Build history of the part. All positions in model axes, mm. A direction names the side the tool comes from. Round coordinates to 2 decimals unless told otherwise and drop trailing zeros. Order: outer loops, then holes, each group sorted by start corner. A loop starts at its lowest first (then second) coordinate and runs counter-clockwise, first axis right, second up. Notation, with made-up numbers: M 19.5,67.5 L 78.5,67.5 A21 cw 78.5,88.5 Z; hole C 36.25,58.5 d5. An arc over 180 degrees is marked long. Use CSV: the item, a comma, the result in double quotes.
from build123d import *

# Parameters (mm, degrees)
F1_DEPTH = 5
F2_R     = 2
F3_R     = 2.224598
F4_DEPTH = 35.001


with BuildPart() as f1:
    # F0 (on Front) → F1 (new body, symmetric)
    with BuildSketch(Plane.XZ):
        Polygon((53.206599, 9.36247), (53.206599, 39.36247), (54.706599, 39.36247), (54.706599, 29.36247), (59.706599, 29.36247), (59.706599, 44.36247), (48.206599, 44.36247), (48.206599, 9.36247), align=None)
    extrude(amount=F1_DEPTH, both=True)

    # F2
    f2_edges = [f1.edges().sort_by_distance(p)[0] for p in [
        (59.706599, 0, 44.36247),
        (53.956599, 5, 44.36247),
        (53.956599, -5, 44.36247),
        (48.206599, 0, 44.36247),
    ]]
    fillet(f2_edges, radius=F2_R)

    # F3 (on face) → F4 (cut, through all)
    with BuildSketch(Plane.XY.offset(44.36247)):
        with Locations((53.791892, 0)):
            Circle(F3_R)
    extrude(amount=-F4_DEPTH, mode=Mode.SUBTRACT)


solid = f1.part
(1) Wall check: line 1 (X direction, y = 3.25, z = 33); line 2 (X direction, y = 0, z = 30.5); line 3 (X direction, y = -4, z = 17). Give the ranges that are in metal, low to high. Write a range as from..to.
Answer block:
line 1,"x = 48.21..53.21, 54.71..59.71"
line 2,"x = 48.21..51.57, 56.02..59.71"
line 3,"x = 48.21..53.21"
(2) Tool access for faces 1 (the face through (54, 3, 39.362)), 2 (the face through (56, -1, 44.362)): list every direction of +Z, -Z, +X, -X, +Y, -Y with a clear straight run to the whole face (end or side of a thin tool).
Answer block:
face 1,"-Z, +Y, -Y"
face 2,"+Z, +X, -X, +Y, -Y"
(3) Cut at A-A, the plane z = 31. Give the cut face in (x, y).
Answer block:
outline,"M 48.21,-5 L 53.21,-5 L 53.21,-2.15 A2.22 cw 53.21,2.15 L 53.21,5 L 48.21,5 Z; M 54.71,-5 L 59.71,-5 L 59.71,5 L 54.71,5 L 54.71,2.03 A2.22 cw 54.71,-2.03 Z"
(4) Cut at B-B, the plane y = 0.5. Give the cut face in (x, z), and give its area (3 significant figures).
Answer block:
outline,"M 48.21,9.36 L 51.62,9.36 L 51.62,44.36 L 50.21,44.36 A2 ccw 48.21,42.36 Z; M 55.96,29.36 L 59.71,29.36 L 59.71,42.36 A2 ccw 57.71,44.36 L 55.96,44.36 Z"
area,"174 mm²"
(5) Cut at C-C, the plane x = 52.5. Give the cut face in (y, z), and give its area (3 significant figures).
Answer block:
outline,"M -5,9.36 L -1.81,9.36 L -1.81,44.36 L -3,44.36 A2 ccw -5,42.36 Z; M 1.81,9.36 L 5,9.36 L 5,42.36 A2 ccw 3,44.36 L 1.81,44.36 Z"
area,"222 mm²"
(6) Drop flat-ended pins along their axis: pin 1 (5 mm diameter, centred on y = 0.5, z = 20, fed in from +X); pin 2 (1 mm diameter, centred on x = 55.5, y = -2, fed in from -Z). Give the stop position or say it passes through.
Answer block:
pin 1,"stops at x = 53.21"
pin 2,"stops at z = 29.36"
(7) Cut at D-D, the plane z = 21. Give the cut face in (x, y).
Answer block:
outline,"M 48.21,-5 L 53.21,-5 L 53.21,-2.15 A2.22 cw 53.21,2.15 L 53.21,5 L 48.21,5 Z"
(8) Two-plate mould, pull along X, no slides. Class faces 3 (the face through (59.707, 0, 36)), 4 (the face through (57, 0, 29.362)), 5 (the face through (54.707, 3, 34)): released by +X, released by -X, zero draft, split by the parting line, or undercut.
Answer block:
face 3,"released by +X"
face 4,"zero draft"
face 5,"undercut"
